Verification items for the finished model (mm, model axes). Round coordinates to 2 decimals unless told otherwise and drop trailing zeros. Write each loop counter-clockwise with the first axis right and the second up, starting at its lowest first coordinate (ties: lowest second). Pieces come first, ordered by that corner, then holes. Notation, with made-up numbers: M 0,71 L 43,71 A20 ccw 43,90 Z; hole C 72,20.5 d7. An arc over 180 degrees is marked long. One line per item, written item: value. Start each with the question number.
Item 1: Section check A-A, the plane z = 33. Record the cut outline in (x, y), then the cut area to 3 significant figures.
Item 2: Thickness scan on probe 1 along Y at (x, z) = (15.5, 57); probe 2 along Z at (x, y) = (25, 17); probe 3 along Y at (x, z) = (50.5, 25.5). Record the ranges inside material, lowest first. Write a range as from..to.
Item 3: Section check B-B, the plane x = 17.5. Record the cut outline in (y, z), then the cut area to 3 significant figures.
Item 4: Gauge pin test, flat end, axial feed: pin 1 (10 mm diameter, centred on x = 37.5, z = 52.5, fed in from -Y). Record the tip position at first contact, or that the pin passes through.
from build123d import *

# Parameters (mm, degrees)
F0_W     = 60
F0_H     = 60
F1_DEPTH = 60
F4_DEPTH = 34.6420161514


with BuildPart() as f1:
    # F0 (on Top) → F1 (new body)
    with BuildSketch(Plane.XY):
        with Locations((30, 30)):
            Rectangle(F0_W, F0_H)
    extrude(amount=F1_DEPTH)

    # F3 (on 3pt) → F4 (cut, through all)
    with BuildSketch(Plane(origin=(20, -20, 20), x_dir=(0.8164965809, 0.4082482905, -0.4082482905), z_dir=(0.5773502692, -0.5773502692, 0.5773502692))):
        Polygon((48.9897948557, 84.8528137424), (-24.4948974278, 42.4264068712), (48.9897948557, 0), align=None)
    extrude(amount=F4_DEPTH, mode=Mode.SUBTRACT)


solid = f1.part
Response values:
1. outline: M 0,0 L 27,0 L 60,33 L 60,60 L 0,60 Z
1. area: 3,060 mm2
2. probe 1: y = 12.5..60
2. probe 2: z = 0..52
2. probe 3: y = 16..60
3. outline: M 0,0 L 60,0 L 60,60 L 17.5,60 L 0,42.5 Z
3. area: 3,450 mm2
4. pin 1: stops at y = 22.93
